Input: part model. Units: mm. Frame: model coordinates. A direction names the side the tool comes from. Coordinates: 2 decimals unless noted, no trailing zeros. Order: outer loops, then holes, each group sorted by start corner. A loop starts at its lowest first (then second) coordinate and runs counter-clockwise, first axis right, second up. Notation, with made-up numbers: (28.5, 0) -> (77.5, 0) arc R30 ccw to (77.5, 27) -> close; hole circle Ø9 at (-11.75, 23.25). An arc over 180 degrees is marked (long way). Use CSV: the item, a comma, the result in double quotes. Start each with the question number.
```python
from build123d import *

# Parameters (mm, degrees)
EXTRUDE_1_DEPTH          = 20
FILLET_1_R               = 3
CUT_EXTRUDE_1_DEPTH      = 75.269642706
CUT_EXTRUDE_1_DEPTH_BACK = 75.269642706
SKETCH_2_R               = 2.3
SKETCH_3_W               = 20
SKETCH_3_H               = 35.3
EXTRUDE_2_DEPTH          = 4
SKETCH_4_W               = 5
SKETCH_4_H               = 42
EXTRUDE_3_DEPTH          = 38.5
EXTRUDE_4_DEPTH          = 6.7
CUT_EXTRUDE_2_REACH      = 119.861
SKETCH_6_R               = 11.5
SKETCH_6_R_2             = 1.7
FILLET_2_R               = 7
CUT_EXTRUDE_3_REACH      = 108.144
SKETCH_9_R               = 3.5
SKETCH_10_W              = 11.60500139
SKETCH_10_H              = 6
EXTRUDE_6_DEPTH          = 5


with BuildPart() as part:
    # 草图1 → 凸台-拉伸1 (new body)
    with BuildSketch(Plane.XY):
        with BuildLine():
            Line((54.2, 3.8), (54.2, 0.3))
            Line((54.2, 0.3), (70.99499861, 0.3))
            Line((70.99499861, 0.3), (70.99499861, 4.3))
            Line((70.99499861, 4.3), (63.612861565, 4.3))
            ThreePointArc((63.612861565, 4.3), (60.381762681, 5.244310136), (58.167716939, 7.78))
            ThreePointArc((58.167716939, 7.78), (50, 13), (41.832283061, 7.78))
            ThreePointArc((41.832283061, 7.78), (39.618237319, 5.244310136), (36.387138435, 4.3))
            Line((36.387138435, 4.3), (-36.387138435, 4.3))
            ThreePointArc((-36.387138435, 4.3), (-39.618237319, 5.244310136), (-41.832283061, 7.78))
            ThreePointArc((-41.832283061, 7.78), (-50, 13), (-58.167716939, 7.78))
            ThreePointArc((-58.167716939, 7.78), (-60.381762681, 5.244310136), (-63.612861565, 4.3))
            Line((-63.612861565, 4.3), (-70.99499861, 4.3))
            Line((-70.99499861, 4.3), (-70.99499861, 0.3))
            Line((-70.99499861, 0.3), (-54.2, 0.3))
            Line((-54.2, 0.3), (-54.2, 3.8))
            ThreePointArc((-54.2, 3.8), (-50, 8), (-45.8, 3.8))
            Line((-45.8, 3.8), (-45.8, 0.3))
            Line((-45.8, 0.3), (45.8, 0.3))
            Line((45.8, 0.3), (45.8, 3.8))
            ThreePointArc((45.8, 3.8), (50, 8), (54.2, 3.8))
        make_face()
    extrude(amount=EXTRUDE_1_DEPTH)

    # 圆角1
    fillet_1_edges = [part.edges().sort_by_distance(p)[0] for p in [
        (70.99499861, 2.3, 20),
        (-70.99499861, 2.3, 0),
        (70.99499861, 2.3, 0),
        (-70.99499861, 2.3, 20),
    ]]
    fillet(fillet_1_edges, radius=FILLET_1_R)

    # 草图2 → 切除-拉伸1 (cut, two sides: drawn at the far end of the back side and taken through both)
    with BuildSketch(Plane(origin=(0, 4.3, 0), x_dir=(1, 0, 0), z_dir=(0, 1, 0)).offset(-CUT_EXTRUDE_1_DEPTH_BACK)):
        with Locations(Location((66.39499861, -10, 0), (0, 0, 270))):
            Circle(SKETCH_2_R)
        with Locations(Location((33.60500139, -10, 0), (0, 0, 90))):
            Circle(SKETCH_2_R)
        with Locations(Location((-33.60500139, -10, 0), (0, 0, 270))):
            Circle(SKETCH_2_R)
        with Locations((-66.39499861, -10)):
            Circle(SKETCH_2_R)
    extrude(amount=CUT_EXTRUDE_1_DEPTH + CUT_EXTRUDE_1_DEPTH_BACK, mode=Mode.SUBTRACT)

    # 草图3 → 凸台-拉伸2 (add)
    with BuildSketch(Plane.XY.offset(20)):
        with Locations((14, -13.35)):
            Rectangle(SKETCH_3_W, SKETCH_3_H)
    extrude(amount=EXTRUDE_2_DEPTH)

    # 草图4 → 凸台-拉伸3 (add)
    with BuildSketch(Plane.XY.offset(24)):
        with Locations((6.5, -10)):
            Rectangle(SKETCH_4_W, SKETCH_4_H)
    extrude(amount=EXTRUDE_3_DEPTH)

    # 草图5 → 凸台-拉伸4 (add)
    with BuildSketch(Plane(origin=(0, 4.3, 0), x_dir=(1, 0, 0), z_dir=(0, 1, 0))):
        Polygon((4, -13), (4, -24), (24, -24), (24, 0), (4, 0), align=None)
    extrude(amount=EXTRUDE_4_DEPTH)

    # 草图6 → 切除-拉伸2 (cut, up to next)
    with BuildSketch(Plane(origin=(24, 0, 0), x_dir=(0, 0, -1), z_dir=(1, 0, 0)), mode=Mode.PRIVATE) as cut_extrude_2_sk1:
        with Locations(Location((-41.25, -10, 0), (0, 0, 90))):
            Circle(SKETCH_6_R)
    cut_extrude_2_tool1 = extrude(cut_extrude_2_sk1.sketch, amount=-CUT_EXTRUDE_2_REACH, mode=Mode.PRIVATE) & part.part
    # 草图6 → 切除-拉伸2 (cut, up to next)
    with BuildSketch(Plane(origin=(24, 0, 0), x_dir=(0, 0, -1), z_dir=(1, 0, 0)), mode=Mode.PRIVATE) as cut_extrude_2_sk2:
        with Locations(Location((-25.75, 5.5, 0), (0, 0, 90))):
            Circle(SKETCH_6_R_2)
    cut_extrude_2_tool2 = extrude(cut_extrude_2_sk2.sketch, amount=-CUT_EXTRUDE_2_REACH, mode=Mode.PRIVATE) & part.part
    # 草图6 → 切除-拉伸2 (cut, up to next)
    with BuildSketch(Plane(origin=(24, 0, 0), x_dir=(0, 0, -1), z_dir=(1, 0, 0)), mode=Mode.PRIVATE) as cut_extrude_2_sk3:
        with Locations(Location((-25.75, -25.5, 0), (0, 0, 90))):
            Circle(SKETCH_6_R_2)
    cut_extrude_2_tool3 = extrude(cut_extrude_2_sk3.sketch, amount=-CUT_EXTRUDE_2_REACH, mode=Mode.PRIVATE) & part.part
    # 草图6 → 切除-拉伸2 (cut, up to next)
    with BuildSketch(Plane(origin=(24, 0, 0), x_dir=(0, 0, -1), z_dir=(1, 0, 0)), mode=Mode.PRIVATE) as cut_extrude_2_sk4:
        with Locations(Location((-56.75, -25.5, 0), (0, 0, 90))):
            Circle(SKETCH_6_R_2)
    cut_extrude_2_tool4 = extrude(cut_extrude_2_sk4.sketch, amount=-CUT_EXTRUDE_2_REACH, mode=Mode.PRIVATE) & part.part
    # 草图6 → 切除-拉伸2 (cut, up to next)
    with BuildSketch(Plane(origin=(24, 0, 0), x_dir=(0, 0, -1), z_dir=(1, 0, 0)), mode=Mode.PRIVATE) as cut_extrude_2_sk5:
        with Locations(Location((-56.75, 5.5, 0), (0, 0, 90))):
            Circle(SKETCH_6_R_2)
    cut_extrude_2_tool5 = extrude(cut_extrude_2_sk5.sketch, amount=-CUT_EXTRUDE_2_REACH, mode=Mode.PRIVATE) & part.part
    add(cut_extrude_2_tool1.solids().sort_by_distance((24, -10, 41.25))[0], mode=Mode.SUBTRACT)
    add(cut_extrude_2_tool2.solids().sort_by_distance((24, 5.5, 25.75))[0], mode=Mode.SUBTRACT)
    add(cut_extrude_2_tool3.solids().sort_by_distance((24, -25.5, 25.75))[0], mode=Mode.SUBTRACT)
    add(cut_extrude_2_tool4.solids().sort_by_distance((24, -25.5, 56.75))[0], mode=Mode.SUBTRACT)
    add(cut_extrude_2_tool5.solids().sort_by_distance((24, 5.5, 56.75))[0], mode=Mode.SUBTRACT)

    # 圆角2
    # the kernel refuses this fillet: 7 mm, written as the material it adds along each edge
    with BuildSketch(Plane(origin=(4, 4.3, 0), x_dir=(0, 1, 0), z_dir=(0, 0, 1))) as fillet_2_piece_1:
        with BuildLine():
            CenterArc((7, 6.993568474), FILLET_2_R, 180, 87.543714276)
            Line((0, 6.993568474), (-0.14, 6.993568474))
            Line((-0.14, 6.993568474), (-0.14, 0))
            Line((-0.14, 0), (0, -0.14))
            ThreePointArc((0, -0.14), (3.35, -0.14), (6.694, -0.139871369))
            Line((6.694, -0.139871369), (6.7, 0))
        make_face()
    extrude(amount=20)
    with BuildSketch(Plane(origin=(24, 4.3, 20), x_dir=(1, 0, 0), z_dir=(0, 0, -1))) as fillet_2_piece_2:
        with BuildLine():
            CenterArc((6.993568474, -7), FILLET_2_R, 90, 87.543714276)
            Line((0, -6.7), (-0.139871369, -6.694))
            ThreePointArc((-0.139871369, -6.694), (-0.14, -3.35), (-0.14, 0))
            Line((-0.14, 0), (0, 0.14))
            Line((0, 0.14), (6.993568474, 0.14))
            Line((6.993568474, 0.14), (6.993568474, 0))
        make_face()
    extrude(amount=20)

    # 草图9 → 切除-拉伸3 (cut, up to next)
    with BuildSketch(Plane(origin=(9, 0, 0), x_dir=(0, 0, -1), z_dir=(1, 0, 0)), mode=Mode.PRIVATE) as cut_extrude_3_sk1:
        with Locations((-25.75, 5.5)):
            Circle(SKETCH_9_R)
    cut_extrude_3_tool1 = extrude(cut_extrude_3_sk1.sketch, amount=CUT_EXTRUDE_3_REACH, mode=Mode.PRIVATE) & part.part
    # 草图9 → 切除-拉伸3 (cut, up to next)
    with BuildSketch(Plane(origin=(9, 0, 0), x_dir=(0, 0, -1), z_dir=(1, 0, 0)), mode=Mode.PRIVATE) as cut_extrude_3_sk2:
        with Locations((-25.75, -25.5)):
            Circle(SKETCH_9_R)
    cut_extrude_3_tool2 = extrude(cut_extrude_3_sk2.sketch, amount=CUT_EXTRUDE_3_REACH, mode=Mode.PRIVATE) & part.part
    add(cut_extrude_3_tool1.solids().sort_by_distance((9, 5.5, 25.75))[0], mode=Mode.SUBTRACT)
    add(cut_extrude_3_tool2.solids().sort_by_distance((9, -25.5, 25.75))[0], mode=Mode.SUBTRACT)

    # 草图10 → 凸台-拉伸6 (add)
    with BuildSketch(Plane.XZ.offset(-0.3)):
        with Locations((17.802500695, 10)):
            Rectangle(SKETCH_10_W, SKETCH_10_H)
        with Locations((-17.802500695, 10)):
            Rectangle(SKETCH_10_W, SKETCH_10_H)
    extrude(amount=EXTRUDE_6_DEPTH)


solid = part.part
```
1. Section D-D on z = 41.25. Return loops of the section in (x, y), then the cut area to 3 significant figures.
2. Section C-C on y = -25.5. Return loops of the section in (x, z).
3. Access query for faces 1 (the face through (39.66, 5.27, 9.86)), 2 (the face through (62, 0.3, 10)), 3 (the face through (54.2, 2, 10)). Directions: +Z, -Z, +X, -X, +Y, -Y. A direction counts if a zero-diameter tool reaches every point of the face in a straight line with its end or side. Return the directions, or none.
4. Section B-B on z = 56.75. Return loops of the section in (x, y).
5. Pull-direction query (X, two-part tool) for faces 4 (the face through (-12, -2, 10)), 5 (the face through (4, -1, 50)), 6 (the face through (16, -30, 24)); classes: released by +X, released by -X, zero draft, split by the parting line, or undercut.
6. Contact query for flat-ended pins moving along their axis: P1, Ø4, axis at x = 17.5, y = -3, coming from the -Z side; P2, Ø6, axis at x = 33.61, z = 10, coming from the -Y side; P3, Ø4, axis at x = 46.5, y = 9.5, coming from the +Z side; P4, Ø2, axis at x = -55.5, z = 22, coming from the +Y side. Output: stop coordinate, or through.
7. Section A-A on y = -10. Return loops of the section in (x, z).
8. Material intervals for line 1 along Y through (x, z) = (7, 41); line 2 along Y through (x, z) = (6, 56); line 3 along X through (y, z) = (9, 13), sorted ascending.
Values follow:
1,outline,"(4, -31) -> (9, -31) -> (9, -21.5) -> (4, -21.5) -> close; (4, 1.5) -> (9, 1.5) -> (9, 11) -> (4, 11) -> close"
1,area,"95.0 mm2"
2,outline,"(4, 20) -> (24, 20) -> (24, 22.25) -> (9, 22.25) -> (9, 24.05) -> (4, 24.05) -> close; (4, 27.45) -> (9, 27.45) -> (9, 55.05) -> (4, 55.05) -> close; (4, 58.45) -> (9, 58.45) -> (9, 62.5) -> (4, 62.5) -> close"
3,face 1,"+Z, -Z, +Y"
3,face 2,"+Z, -Z, +X, -Y"
3,face 3,"+Z, -Z, -Y"
4,outline,"(4, -31) -> (9, -31) -> (9, -27.2) -> (4, -27.2) -> close; (4, -23.8) -> (9, -23.8) -> (9, 3.8) -> (4, 3.8) -> close; (4, 7.2) -> (9, 7.2) -> (9, 11) -> (4, 11) -> close"
5,face 4,"undercut"
5,face 5,"released by -X"
5,face 6,"zero draft"
6,P1,"stops at z = 7"
6,P2,"stops at y = 0.3"
6,P3,"stops at z = 20"
6,P4,"passes through"
7,outline,"(4, 20) -> (24, 20) -> (24, 24) -> (9, 24) -> (9, 29.75) -> (4, 29.75) -> close; (4, 52.75) -> (9, 52.75) -> (9, 62.5) -> (4, 62.5) -> close"
8,line 1,"y = -31 to -21.5, 1.5 to 11"
8,line 2,"y = -31 to -27.03, -23.97 to 3.97, 7.03 to 11"
8,line 3,"x = -57.48 to -42.52, 3.62 to 24.38, 42.52 to 57.48"
